Work out the finished part from the listing and answer in its coordinate system (mm). Give positions to 0.01 mm unless a question says otherwise; leave off trailing zeros. Loops run counter-clockwise (first coordinate to the right, second up) from the corner with the lowest first, then second, coordinate; pieces in that order, holes last. Notation, with made-up numbers: (36, 59) - (61, 59) arc R19 cw to (61, 78) - close; hole circle Ø8 at (3.5, 64). An arc over 180 degrees is marked (long way). One line per question, with ' | ' between items. Start each with the question number.
1. Section A-A (x = -19) is taken. Determine the outline of the cut face in (y, z).
2. Section B-B (y = -0.15) is taken. Determine the outline of the cut face in (x, z), plus the area to 3 significant figures.
3. Find the intervals of material crossed by line 1 (Z direction, x = 4.5, y = -1.35); line 2 (X direction, y = 1.4, z = 14); line 3 (Z direction, x = 32, y = 1.2), in increasing order.
4. Each of these flat-tipped pins is pushed along its axis until it touches: pin 1 (1.5 mm diameter, centred on x = -10, y = 0, fed in from -Z); pin 2 (3 mm diameter, centred on x = 23, y = 1.5, fed in from +Z). Where does it stop, or does it pass through?
5. Section C-C (z = 27) is taken. Determine the outline of the cut face in (x, y).
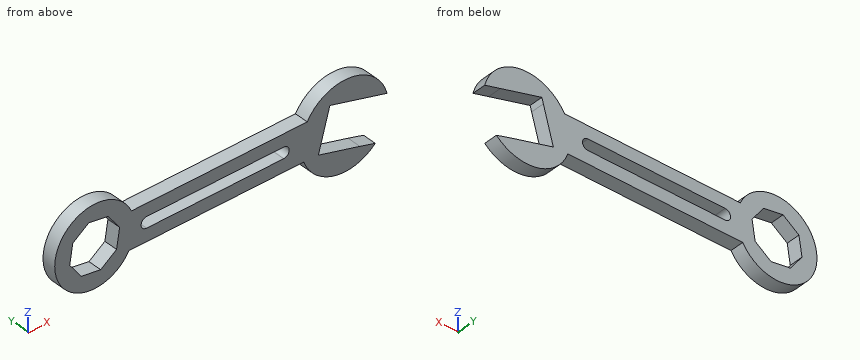
from build123d import *

# Parameters (mm, degrees)
F1_DEPTH = 2.54


with BuildPart() as f1:
    # F0 (on Front) → F1 (new body, symmetric)
    with BuildSketch(Plane.XZ):
        with BuildLine():
            Line((-34.314002, 9.582906), (-34.314002, 21.31113))
            ThreePointArc((-34.314002, 21.31113), (-62.691893, 16.413153), (-35.19322, 7.862254))
            ThreePointArc((-35.19322, 7.862254), (-34.725519, 8.708226), (-34.314002, 9.582906))
        make_face()
        Polygon((-42.942699, 23.557279), (-38.663793, 17.666949), (-39.803242, 10.476214), (-45.693572, 6.197308), (-52.884307, 7.336757), (-57.163212, 13.227087), (-56.023764, 20.417822), (-50.133434, 24.696727), align=None, mode=Mode.SUBTRACT)
        with BuildLine():
            Line((30.832, 21.31113), (-34.314002, 21.31113))
            Line((-34.314002, 21.31113), (-34.314002, 9.582906))
            ThreePointArc((-34.314002, 9.582906), (-34.725519, 8.708226), (-35.19322, 7.862254))
            Line((-35.19322, 7.862254), (-34.314002, 7.862254))
            Line((-34.314002, 7.862254), (29.576525, 7.862254))
            ThreePointArc((29.576525, 7.862254), (28.726842, 14.724611), (30.832, 21.31113))
        make_face()
        with BuildLine():
            ThreePointArc((-28.677113, 12.598262), (-30.70935, 14.630499), (-28.677113, 16.662735))
            Line((-28.677113, 16.662735), (22.128796, 16.662735))
            ThreePointArc((22.128796, 16.662735), (24.161033, 14.630499), (22.128796, 12.598262))
            Line((22.128796, 12.598262), (-28.677113, 12.598262))
        make_face(mode=Mode.SUBTRACT)
        with BuildLine():
            ThreePointArc((60.391538, 17.164629), (47.006746, 29.182375), (30.832, 21.31113))
            ThreePointArc((30.832, 21.31113), (28.726842, 14.724611), (29.576525, 7.862254))
            ThreePointArc((29.576525, 7.862254), (41.1317, -2.468564), (56.052909, 1.727312))
            Line((56.052909, 1.727312), (50.318425, 3.422388))
            Line((50.318425, 3.422388), (34.963898, 7.677261))
            Line((34.963898, 7.677261), (38.663793, 21.029043))
            Line((38.663793, 21.029043), (39.218771, 23.031787))
            Line((39.218771, 23.031787), (54.573298, 18.776914))
            Line((54.573298, 18.776914), (60.391538, 17.164629))
        make_face()
    extrude(amount=F1_DEPTH, both=True)


solid = f1.part
Conclusion:
1) outline: (-2.54, 7.86) - (2.54, 7.86) - (2.54, 12.6) - (-2.54, 12.6) - close; (-2.54, 16.66) - (2.54, 16.66) - (2.54, 21.31) - (-2.54, 21.31) - close
2) outline: (-35.19, 7.86) - (29.58, 7.86) arc R16.11 ccw to (56.05, 1.73) - (50.32, 3.42) - (34.96, 7.68) - (39.22, 23.03) - (60.39, 17.16) arc R16.11 ccw to (30.83, 21.31) - (-34.31, 21.31) arc R14.81 ccw (long way) to start; hole (-57.16, 13.23) - (-52.88, 7.34) - (-45.69, 6.2) - (-39.8, 10.48) - (-38.66, 17.67) - (-42.94, 23.56) - (-50.13, 24.7) - (-56.02, 20.42) - close; hole (-28.68, 12.6) - (22.13, 12.6) arc R2.03 ccw to (22.13, 16.66) - (-28.68, 16.66) arc R2.03 ccw to start | area: 1,500 mm²
3) line 1: 7.86 to 12.6, 16.66 to 21.31 | line 2: -62.65 to -57.04, -39.24 to -30.61, 24.06 to 36.72 | line 3: 3.4 to 23.05
4) pin 1: z = 7.86 | pin 2: z = 21.31
5) outline: (-57.18, -2.54) - (-38.65, -2.54) - (-38.65, 2.54) - (-57.18, 2.54) - close; (36.41, -2.54) - (53.13, -2.54) - (53.13, 2.54) - (36.41, 2.54) - close
